```python
from build123d import *

# Parameters (mm, degrees)
F0_W     = 39
F0_H     = 39
F1_DEPTH = 2
F2_DEPTH = 35
F3_SIZE2 = 10
F3_SIZE  = 1.6
F4_DEPTH = 30
F5_SIZE2 = 3
F5_SIZE  = 0.3
F0_W_2   = 12.1088270918
F0_H_2   = 1
F0_W_3   = 1
F0_H_3   = 12.5
F6_DEPTH = 30
F7_R     = 3
F8_R     = 1


with BuildPart() as f1:
    # F0 (on Top) → F1 (new body)
    with BuildSketch(Plane.XY):
        Rectangle(F0_W, F0_H)
        with BuildLine():
            Line((-16, -11), (-16, 11))
            ThreePointArc((-16, 11), (-14.5355339059, 14.5355339059), (-11, 16))
            Line((-11, 16), (11, 16))
            ThreePointArc((11, 16), (14.5355339059, 14.5355339059), (16, 11))
            Line((16, 11), (16, -11))
            ThreePointArc((16, -11), (14.5355339059, -14.5355339059), (11, -16))
            Line((11, -16), (-11, -16))
            ThreePointArc((-11, -16), (-14.5355339059, -14.5355339059), (-16, -11))
        make_face(mode=Mode.SUBTRACT)
        with BuildLine():
            ThreePointArc((-11, 16), (-14.5355339059, 14.5355339059), (-16, 11))
            Line((-16, 11), (-16, -11))
            ThreePointArc((-16, -11), (-14.5355339059, -14.5355339059), (-11, -16))
            Line((-11, -16), (11, -16))
            ThreePointArc((11, -16), (14.5355339059, -14.5355339059), (16, -11))
            Line((16, -11), (16, 11))
            ThreePointArc((16, 11), (14.5355339059, 14.5355339059), (11, 16))
            Line((11, 16), (-11, 16))
        make_face()
        with BuildLine():
            Line((-14, -11), (-14, 11))
            ThreePointArc((-14, 11), (-13.1213203436, 13.1213203436), (-11, 14))
            Line((-11, 14), (11, 14))
            ThreePointArc((11, 14), (13.1213203436, 13.1213203436), (14, 11))
            Line((14, 11), (14, -11))
            ThreePointArc((14, -11), (13.1213203436, -13.1213203436), (11, -14))
            Line((11, -14), (-11, -14))
            ThreePointArc((-11, -14), (-13.1213203436, -13.1213203436), (-14, -11))
        make_face(mode=Mode.SUBTRACT)
    extrude(amount=F1_DEPTH)

    # F0 (on Top) → F2 (join)
    with BuildSketch(Plane.XY):
        with BuildLine():
            ThreePointArc((-11, 16), (-14.5355339059, 14.5355339059), (-16, 11))
            Line((-16, 11), (-16, -11))
            ThreePointArc((-16, -11), (-14.5355339059, -14.5355339059), (-11, -16))
            Line((-11, -16), (11, -16))
            ThreePointArc((11, -16), (14.5355339059, -14.5355339059), (16, -11))
            Line((16, -11), (16, 11))
            ThreePointArc((16, 11), (14.5355339059, 14.5355339059), (11, 16))
            Line((11, 16), (-11, 16))
        make_face()
        with BuildLine():
            Line((-14, -11), (-14, 11))
            ThreePointArc((-14, 11), (-13.1213203436, 13.1213203436), (-11, 14))
            Line((-11, 14), (11, 14))
            ThreePointArc((11, 14), (13.1213203436, 13.1213203436), (14, 11))
            Line((14, 11), (14, -11))
            ThreePointArc((14, -11), (13.1213203436, -13.1213203436), (11, -14))
            Line((11, -14), (-11, -14))
            ThreePointArc((-11, -14), (-13.1213203436, -13.1213203436), (-14, -11))
        make_face(mode=Mode.SUBTRACT)
    extrude(amount=F2_DEPTH)

    # F3
    f3_edges = [f1.edges().sort_by_distance(p)[0] for p in [
        (0, -16, 35),
        (14.535534, -14.535534, 35),
        (16, 0, 35),
        (14.535534, 14.535534, 35),
        (0, 16, 35),
        (-14.535534, 14.535534, 35),
        (-16, 0, 35),
        (-14.535534, -14.535534, 35),
    ]]
    f3_side = f1.faces().sort_by_distance((-14.215534, 14.215534, 35))[0]
    chamfer(f3_edges, length=F3_SIZE, length2=F3_SIZE2, reference=f3_side)

    # F0 (on Top) → F4 (join)
    with BuildSketch(Plane.XY):
        with BuildLine():
            ThreePointArc((-11, 14), (-13.1213203436, 13.1213203436), (-14, 11))
            Line((-14, 11), (-14, -11))
            ThreePointArc((-14, -11), (-13.1213203436, -13.1213203436), (-11, -14))
            Line((-11, -14), (11, -14))
            ThreePointArc((11, -14), (13.1213203436, -13.1213203436), (14, -11))
            Line((14, -11), (14, 11))
            ThreePointArc((14, 11), (13.1213203436, 13.1213203436), (11, 14))
            Line((11, 14), (-11, 14))
        make_face()
        Polygon((-12.6088270918, 0.5), (-12.6088270918, 13), (-0.5, 13), (0.5, 13), (12.6088270918, 13), (12.6088270918, 0.5), (12.6088270918, -0.5), (12.6088270918, -13), (0.5, -13), (-0.5, -13), (-12.6088270918, -13), (-12.6088270918, -0.5), align=None, mode=Mode.SUBTRACT)
    extrude(amount=F4_DEPTH)

    # F5
    f5_edges = [f1.edges().sort_by_distance(p)[0] for p in [
        (0, 14, 35),
        (13.12132, 13.12132, 35),
        (14, 0, 35),
        (13.12132, -13.12132, 35),
        (0, -14, 35),
        (-13.12132, -13.12132, 35),
        (-14, 0, 35),
        (-13.12132, 13.12132, 35),
    ]]
    f5_side = f1.faces().sort_by_distance((0, -14.359271, 35))[0]
    chamfer(f5_edges, length=F5_SIZE, length2=F5_SIZE2, reference=f5_side)

    # F0 (on Top) → F6 (join)
    with BuildSketch(Plane.XY):
        with Locations((6.5544135459, 0)):
            Rectangle(F0_W_2, F0_H_2)
        with Locations((0, -6.75)):
            Rectangle(F0_W_3, F0_H_3)
        with Locations((-6.5544135459, 0)):
            Rectangle(F0_W_2, F0_H_2)
        Rectangle(F0_W_3, F0_H_2)
        with Locations((0, 6.75)):
            Rectangle(F0_W_3, F0_H_3)
    extrude(amount=F6_DEPTH)

    # F7
    f7_edges = [f1.edges().sort_by_distance(p)[0] for p in [
        (0, 16, 2),
        (-19.5, 19.5, 1),
        (19.5, 19.5, 1),
        (-19.5, -19.5, 1),
        (19.5, -19.5, 1),
    ]]
    fillet(f7_edges, radius=F7_R)

    # F8
    f8_edges = [f1.edges().sort_by_distance(p)[0] for p in [
        (0, -19.5, 0),
    ]]
    fillet(f8_edges, radius=F8_R)


solid = f1.part
```
Verification items for the finished model (mm, model axes). A direction names the side the tool comes from. Give positions to 0.01 mm unless a question says otherwise; leave off trailing zeros. Loops run counter-clockwise (first coordinate to the right, second up) from the corner with the lowest first, then second, coordinate; pieces in that order, holes last.
1. Section check D-D, the plane z = 7. Enter the section's corners in (x, y).
2. Section check B-B, the plane x = -6. Enter the section's corners in (y, z).
3. Section check C-C, the plane z = 31. Enter the section's corners in (x, y).
4. Go/stop test with flat-tipped pins: pin 1 Ø3.5 at (x, z) = (7, 13.5) entering from -Y; pin 2 Ø6 at (x, y) = (2.5, 4) entering from -Z; pin 3 Ø1.5 at (y, z) = (-12, 21) entering from +X; pin 4 Ø1.6 at (x, z) = (1.5, 31) entering from +Y. Record where each tip stops, or that it passes through.
5. Mould release check, pull along Y, two halves, no side actions. Record for faces 1 (the flat face through (-12.609, -7, 15)), 2 (the flat face through (-15.21, 0.15, 29.93)), 3 (the flat face through (0, -16, 15)): released by +Y, released by -Y, zero draft, split by the parting line, or undercut.
6. Section check A-A, the plane y = -7. Enter the section's corners in (x, z), then the cut area to 3 significant figures.
7. Thickness scan on line 1 (Y direction, x = -11, z = 14.5); line 2 (X direction, y = -11, z = 20); line 3 (Y direction, x = 6, z = 28). Record the ranges inside material, lowest first.
8. Set-up check for faces 4 (the cylindrical face through (-13.14, 13.1, 30.99)), 5 (the cylindrical face through (15, 14, 15)), 6 (the conical face through (13.945, -14.01, 29.93)), 7 (the flat face through (-0.5, 7, 15)), 8 (the cylindrical face through (-19.199, -0.231, 0.285)): record each of +Z, -Z, +X, -X, +Y, -Y from which the full face is reachable in a straight line by a thin tool's end or side.
Geometry says:
1. outline: (-16, -11) arc R5 ccw to (-11, -16) - (11, -16) arc R5 ccw to (16, -11) - (16, 11) arc R5 ccw to (11, 16) - (-11, 16) arc R5 ccw to (-16, 11) - close; hole (-12.61, -13) - (-0.5, -13) - (-0.5, -0.5) - (-12.61, -0.5) - close; hole (-12.61, 0.5) - (-0.5, 0.5) - (-0.5, 13) - (-12.61, 13) - close; hole (0.5, -13) - (12.61, -13) - (12.61, -0.5) - (0.5, -0.5) - close; hole (0.5, 0.5) - (12.61, 0.5) - (12.61, 13) - (0.5, 13) - close
2. outline: (-19.5, 1) arc R1 ccw to (-18.5, 0) - (-13, 0) - (-13, 30) - (-14, 30) - (-14, 32) - (-14.3, 35) - (-14.4, 35) - (-16, 25) - (-16, 5) arc R3 cw to (-19, 2) - (-19.5, 2) - close; (-0.5, 0) - (0.5, 0) - (0.5, 30) - (-0.5, 30) - close; (13, 0) - (18.5, 0) arc R1 ccw to (19.5, 1) - (19.5, 2) - (19, 2) arc R3 cw to (16, 5) - (16, 25) - (14.4, 35) - (14.3, 35) - (14, 32) - (14, 30) - (13, 30) - close
3. outline: (-15.04, -11) arc R4.04 ccw to (-11, -15.04) - (11, -15.04) arc R4.04 ccw to (15.04, -11) - (15.04, 11) arc R4.04 ccw to (11, 15.04) - (-11, 15.04) arc R4.04 ccw to (-15.04, 11) - close; hole (-14, -11) arc R3 ccw to (-11, -14) - (11, -14) arc R3 ccw to (14, -11) - (14, 11) arc R3 ccw to (11, 14) - (-11, 14) arc R3 ccw to (-14, 11) - close
4. pin 1: stops at y = -16
4. pin 2: stops at z = 0
4. pin 3: stops at x = 15.99
4. pin 4: stops at y = 15.17
5. face 1: undercut
5. face 2: zero draft
5. face 3: released by -Y
6. outline: (-19.5, 1) arc R1 ccw to (-18.5, 0) - (-12.61, 0) - (-12.61, 30) - (-14, 30) - (-14, 32) - (-14.3, 35) - (-14.4, 35) - (-16, 25) - (-16, 5) arc R3 cw to (-19, 2) - (-19.5, 2) - close; (-0.5, 0) - (0.5, 0) - (0.5, 30) - (-0.5, 30) - close; (12.61, 0) - (18.5, 0) arc R1 ccw to (19.5, 1) - (19.5, 2) - (19, 2) arc R3 cw to (16, 5) - (16, 25) - (14.4, 35) - (14.3, 35) - (14, 32) - (14, 30) - (12.61, 30) - close
6. area: 254 mm2
7. line 1: y = -16 to -13, -0.5 to 0.5, 13 to 16
7. line 2: x = -16 to -12.61, -0.5 to 0.5, 12.61 to 16
7. line 3: y = -15.52 to -13, -0.5 to 0.5, 13 to 15.52
8. face 4: +Z
8. face 5: +Z, +X, +Y
8. face 6: +Z, +X, -Y
8. face 7: +Z, -Z
8. face 8: -Z, -X, +Y, -Y
